Can you work these out from the model? Positions are in its coordinate system, mm. Round coordinates to 2 decimals unless told otherwise and drop trailing zeros. Order: outer loops, then holes, each group sorted by start corner. A loop starts at its lowest first (then second) coordinate and runs counter-clockwise, first axis right, second up.
from build123d import *

# Parameters (mm, degrees)
EXTRUDE002_DEPTH = 2
SKETCH003_W      = 2
SKETCH003_H      = 35
EXTRUDE001_DEPTH = 45


with BuildPart() as extrude002:
    # Sketch004 (on Face1 of CopyExtrude001) → Extrude002 (new body)
    with BuildSketch(Plane(origin=(0, 0, 0), x_dir=(0, -1, 0), z_dir=(-1, 0, 0))):
        Polygon((-45, 5), (-10, 50), (-45, 50), align=None)
    extrude(amount=-EXTRUDE002_DEPTH)


with BuildPart() as cut001:
    # Sketch003 (on Face1 of CopyCut) → Extrude001 (new body)
    with BuildSketch(Plane.XY.offset(5)):
        with Locations((1, 27.5)):
            Rectangle(SKETCH003_W, SKETCH003_H)
    extrude(amount=EXTRUDE001_DEPTH)

    # Cut001: cut Extrude002
    add(extrude002.part, mode=Mode.SUBTRACT)


solid = cut001.part
(1) Please list where these lines run through material, in increasing order: probe 1 along Y at (x, z) = (0.7, 16.5); probe 2 along Y at (x, z) = (1.2, 16); probe 3 along Z at (x, y) = (1.85, 15).
(2) I'm going to push flat-ended pins straight in: pin 1 Ø6 at (y, z) = (21, 11) entering from -X; pin 2 Ø1 at (x, z) = (1, 14) entering from +Y. Where does each tip first touch, or does it pass through?
(3) I want a section at C-C, the plane x = 1. List the corners of the cut face in (y, z) for me, plus the area to 4 significant figures.
(4) I want a section at A-A, the plane z = 14. List the corners of the cut face in (x, y) for me, plus the area to 3 significant figures.
(5) I want a section at B-B, the plane y = 24. List the corners of the cut face in (x, z) for me, plus the area to 3 significant figures.
Ans:
1. probe 1: y = 10 to 36.06
1. probe 2: y = 10 to 36.44
1. probe 3: z = 5 to 43.57
2. pin 1: stops at x = 0
2. pin 2: stops at y = 38.39
3. outline: (10, 5) - (45, 5) - (10, 50) - close
3. area: 787.5 mm2
4. outline: (0, 10) - (2, 10) - (2, 38) - (0, 38) - close
4. area: 56.0 mm2
5. outline: (0, 5) - (2, 5) - (2, 32) - (0, 32) - close
5. area: 54.0 mm2
